Verification items for this drawing (mm, ordinates from the low corner). Coordinates: 2 decimals unless noted, no trailing zeros. Order: outer loops, then holes, each group sorted by start corner. A loop starts at its lowest first (then second) coordinate and runs counter-clockwise, first axis right, second up. Notation, with made-up numbers: M 41,38.25 L 77,38.25 A6 cw 77,45.25 Z; hole C -12,53 d3. An arc over 180 degrees is marked long. Return JSON: item names as keys, results as strings. Group by question number.
1. Section check C-C, the plane y = 102. Record the cut outline in (x, z).
2. Section check B-B, the plane z = 1.5. Give the number of separate pieces and of enclosed holes in the cut face, plus the area to 3 significant figures.
3. Material ranges on line 1 along Y through (x, z) = (67.5, 0.65) (1 decimal); line 2 along Y through (x, z) = (51, 1.3); line 3 along X through (y, z) = (50, 0.9), recorded low to high.
4. Section check A-A, the plane x = 56. Record the cut outline in (y, z).
5. Section check D-D, the plane x = 24.5. Record the cut outline in (y, z).
6. Gauge pin test, flat ends, axial feed: pin 1 (1.5 mm diameter, centred on y = 13.5, z = 0.5, fed in from -X) (1 decimal); pin 2 (1.5 mm diameter, centred on y = 41.5, z = 0.5, fed in from +X); pin 3 (2.5 mm diameter, centred on x = 55.91, y = 3.75, fed in from +Z); pin 4 (1 mm diameter, centred on y = 64, z = 2, fed in from -X). Record the tip position at first contact, or that the pin passes through.
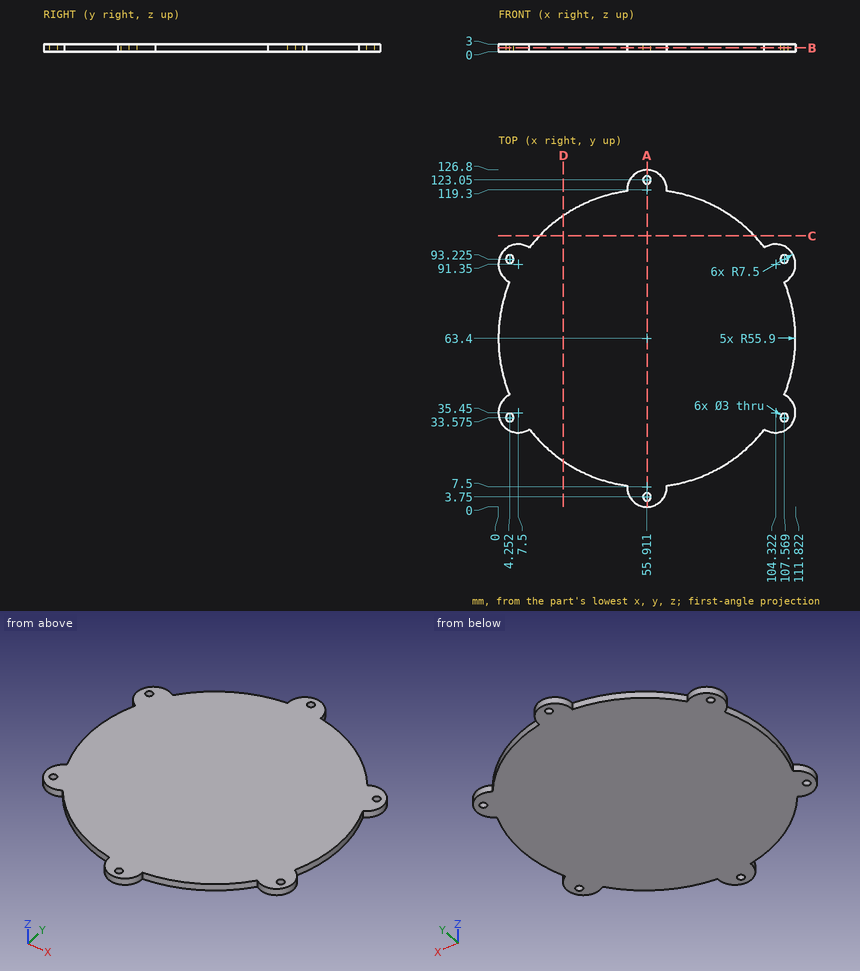
Answers follow:
{
 "1": {"outline": "M 15.48,0 L 96.34,0 L 96.34,3 L 15.48,3 Z"},
 "2": {"separate pieces": "1", "enclosed holes": "6", "area": "10,300 mm^2"},
 "3": {"line 1": "8.7 to 118.1", "line 2": "1.83 to 124.97", "line 3": "1.64 to 110.18"},
 "4": {"outline": "M 0,0 L 2.25,0 L 2.25,3 L 0,3 Z; M 5.25,0 L 121.55,0 L 121.55,3 L 5.25,3 Z; M 124.55,0 L 126.8,0 L 126.8,3 L 124.55,3 Z"},
 "5": {"outline": "M 17.16,0 L 109.64,0 L 109.64,3 L 17.16,3 Z"},
 "6": {"pin 1": "x = 29.3", "pin 2": "x = 109.63", "pin 3": "through", "pin 4": "x = 0.01"}
}
